Autodesk Inventor part; units mm, degrees
ref_plane "YZ Plane" through (0, 0, 0) normal (1, 0, 0) x (0, 1, 0)
ref_plane "XZ Plane" through (0, 0, 0) normal (0, 1, 0) x (-1, 0, 0)
ref_plane "XY Plane" through (0, 0, 0) normal (0, 0, 1) x (1, 0, 0)
sketch "Sketch1" plane through (0, 0, 0) normal (1, 0, 0) x (0, 1, 0)
  line L0 (0, 0) -> (25.4, 0)
  line L1 (25.4, 0) -> (25.4, -25.4)
  line L2 (25.4, -25.4) -> (0, -25.4)
  line L3 (0, -25.4) -> (0, 0)
  line L4 (23.8125, -23.8125) -> (23.8125, -1.5875)
  line L5 (23.8125, -1.5875) -> (1.5875, -1.5875)
  line L6 (1.5875, -1.5875) -> (1.5875, -23.8125)
  line L7 (1.5875, -23.8125) -> (23.8125, -23.8125)
  dimension "d0" = 25.4
  dimension "d1" = 25.4
  dimension "d2" = 1.5875
extrude "Extrusion1" add sketch "Sketch1" along normal blind 1219.2
sketch "Sketch3" plane through (0, 25.4, 0) normal (0, 1, 0) x (1, 0, 0)
  line L0 (0, 23.8125) -> (1219.2, 23.8125)
  line L1 (609.6, 23.8125) -> (609.6, 0) construction
  line L2 (0, 0) -> (1219.2, 0)
  line L3 (609.6, 11.9062) -> (465.3189, 11.9062) construction
  circle A0 centre (304.8, 11.9062) radius 3.175
  circle A1 centre (914.4, 11.9063) radius 3.175
  circle A2 centre (571.5, 11.9063) radius 3.175
  dimension "d10" = 6.35
  dimension "d11" = 304.8
  dimension "d14" = 38.1
extrude "Extrusion3" cut sketch "Sketch3" against normal blind 25.4
sketch "Sketch4" plane through (0, 0, 0) normal (0, 0, 1) x (1, 0, 0)
  line L0 (0, 0) -> (0, 25.4)
  line L1 (0, 12.7) -> (22.1319, 12.7) construction
  circle A0 centre (838.2, 12.7) radius 3.175
  line L2 (0, 0) -> (1219.2, 0)
  line L3 (609.6, 0) -> (609.6, 21.6417) construction
  circle A1 centre (381, 12.7) radius 3.175
  dimension "d15" = 6.35
  dimension "d19" = 228.6
extrude "Extrusion4" cut sketch "Sketch4" against normal blind 25.4
properties part number "Lomg horizontal"
Verification items for the finished model (mm, model axes). A direction names the side the tool comes from. Coordinates: 2 decimals unless noted, no trailing zeros. Loops run counter-clockwise (first coordinate to the right, second up) from the corner with the lowest first, then second, coordinate; pieces in that order, holes last. Notation, with made-up numbers: (70.5, 24.25) - (99.5, 24.25) arc R16 ccw to (99.5, 31.25) - close; hole circle Ø7 at (32, 15.5). An arc over 180 degrees is marked (long way). Put each result on its own line as item: value.
Item 1: Section check A-A (x = 344.5). Enter the section's corners in (y, z).
Conclusion:
outline: (0, -25.4) - (25.4, -25.4) - (25.4, 0) - (0, 0) - close; hole (1.59, -23.81) - (23.81, -23.81) - (23.81, -1.59) - (1.59, -1.59) - close
Item 2: Draft check along Z on faces 1 (the face through (601, 13, -25.4)), 2 (the face through (601, 25.4, -13)), 3 (the face through (601, 23.812, -13)), 4 (the face through (601, 13, 0)). Enter one of: pulls with the +Z half, pulls with the -Z half, needs draft (parallel to the pull), parting line crosses it, or undercut.
Conclusion:
face 1: pulls with the -Z half
face 2: needs draft
face 3: undercut
face 4: pulls with the +Z half
Item 3: Section check B-B (z = -19.25). Enter the section's corners in (x, y).
Conclusion:
outline: (0, 0) - (1219.2, 0) - (1219.2, 1.59) - (0, 1.59) - close; (0, 23.81) - (1219.2, 23.81) - (1219.2, 25.4) - (0, 25.4) - close
Item 4: Set-up check for faces 5 (the face through (601, 1.588, -13)), 6 (the face through (0, 1, -13)): record each of +Z, -Z, +X, -X, +Y, -Y from which the full face is reachable in a straight line by a thin tool's end or side.
Conclusion:
face 5: +X, -X
face 6: +Z, -Z, -X, +Y, -Y
Item 5: Scan lines: line 1 along Y through (x, z) = (1003, -10.75); line 2 along Z through (x, y) = (1158.5, 17.25); line 3 along Z through (x, y) = (304.8, 0.7). Record each from-to range of solid material in increasing order.
Conclusion:
line 1: y = 0 to 1.59, 23.81 to 25.4
line 2: z = -25.4 to -23.81, -1.59 to 0
line 3: z = -25.4 to -15.08, -8.73 to 0
